```python
from build123d import *

# Parameters (mm, degrees)
EXTRUDE_1_DEPTH             = 38
SKETCH_3_R                  = 4.35
EXTRUDE_2_DEPTH             = 288
EXTRUDE_3_DEPTH             = 38
SKETCH_5_W                  = 42
SKETCH_5_H                  = 27.5
PATTERN_LINEAR_1_COUNT      = 2
PATTERN_LINEAR_1_PITCH      = 89
PATTERN_LINEAR_1_COUNT_DIR2 = 2
PATTERN_LINEAR_1_PITCH_DIR2 = 89
PATTERN_LINEAR_2_COUNT      = 2
PATTERN_LINEAR_2_PITCH      = 89
PATTERN_LINEAR_2_COUNT_DIR2 = 2
PATTERN_LINEAR_2_PITCH_DIR2 = 89


with BuildPart() as part:
    # Sketch 1 → Extrude 1 (new body)
    with BuildSketch(Plane(origin=(0, 0, 0), x_dir=(0, 0, -1), z_dir=(1, 0, 0))):
        with BuildLine():
            Line((-52, -57), (52, -57))
            ThreePointArc((52, -57), (55.535533906, -55.535533906), (57, -52))
            Line((57, -52), (57, 52))
            ThreePointArc((57, 52), (55.535533906, 55.535533906), (52, 57))
            Line((52, 57), (-52, 57))
            ThreePointArc((-52, 57), (-55.535533906, 55.535533906), (-57, 52))
            Line((-57, 52), (-57, -52))
            ThreePointArc((-57, -52), (-55.535533906, -55.535533906), (-52, -57))
        make_face()
    extrude(amount=EXTRUDE_1_DEPTH)

    # Sketch 2 → Revolve 1 (revolve)
    with BuildSketch(Plane(origin=(0, 0, 0), x_dir=(1, 0, 0), z_dir=(0, 1, 0))):
        with BuildLine():
            Line((-20, 0), (-20, 23))
            ThreePointArc((-20, 23), (-19.707106781, 23.707106781), (-19, 24))
            Line((-19, 24), (-5, 24))
            Line((-5, 24), (-5, 26.5))
            ThreePointArc((-5, 26.5), (-4.707106781, 27.207106781), (-4, 27.5))
            Line((-4, 27.5), (38, 27.5))
            Line((38, 27.5), (38, 0))
            Line((38, 0), (-20, 0))
        make_face()
    revolve(axis=Axis((38, 0, 0), (-1, 0, 0)))

    # Sketch 3 → Extrude 2 (add)
    with BuildSketch(Plane(origin=(38, 0, 0), x_dir=(0, 0, -1), z_dir=(1, 0, 0))):
        with BuildLine():
            Line((-43.968530717, -33.361928999), (-51.303300859, -40.696699141))
            ThreePointArc((-51.303300859, -40.696699141), (-51.303300859, -51.303300859), (-40.696699141, -51.303300859))
            Line((-40.696699141, -51.303300859), (-33.361928999, -43.968530717))
            ThreePointArc((-33.361928999, -43.968530717), (-32.119521583, -43.390137282), (-30.796446235, -43.747330196))
            ThreePointArc((-30.796446235, -43.747330196), (1.08e-07, -53.5), (30.796446412, -43.747330071))
            ThreePointArc((30.796446412, -43.747330071), (32.119521691, -43.390137291), (33.361928999, -43.968530717))
            Line((33.361928999, -43.968530717), (40.696699141, -51.303300859))
            ThreePointArc((40.696699141, -51.303300859), (51.303300859, -51.303300859), (51.303300859, -40.696699141))
            Line((51.303300859, -40.696699141), (43.968530717, -33.361928999))
            ThreePointArc((43.968530717, -33.361928999), (43.390137282, -32.119521583), (43.747330196, -30.796446235))
            ThreePointArc((43.747330196, -30.796446235), (53.5, 1.08e-07), (43.747330071, 30.796446412))
            ThreePointArc((43.747330071, 30.796446412), (43.390137291, 32.119521691), (43.968530717, 33.361928999))
            Line((43.968530717, 33.361928999), (51.303300859, 40.696699141))
            ThreePointArc((51.303300859, 40.696699141), (51.303300859, 51.303300859), (40.696699141, 51.303300859))
            Line((40.696699141, 51.303300859), (33.361928999, 43.968530717))
            ThreePointArc((33.361928999, 43.968530717), (32.119521583, 43.390137282), (30.796446235, 43.747330196))
            ThreePointArc((30.796446235, 43.747330196), (-1.08e-07, 53.5), (-30.796446412, 43.747330071))
            ThreePointArc((-30.796446412, 43.747330071), (-32.119521691, 43.390137291), (-33.361928999, 43.968530717))
            Line((-33.361928999, 43.968530717), (-40.696699141, 51.303300859))
            ThreePointArc((-40.696699141, 51.303300859), (-51.303300859, 51.303300859), (-51.303300859, 40.696699141))
            Line((-51.303300859, 40.696699141), (-43.968530717, 33.361928999))
            ThreePointArc((-43.968530717, 33.361928999), (-43.390137282, 32.119521583), (-43.747330196, 30.796446235))
            ThreePointArc((-43.747330196, 30.796446235), (-53.5, -1.08e-07), (-43.747330071, -30.796446412))
            ThreePointArc((-43.747330071, -30.796446412), (-43.390137291, -32.119521691), (-43.968530717, -33.361928999))
        make_face()
        with Locations((44.5, 44.5)):
            Circle(SKETCH_3_R, mode=Mode.SUBTRACT)
        with Locations((44.5, -44.5)):
            Circle(SKETCH_3_R, mode=Mode.SUBTRACT)
        with Locations((-44.5, 44.5)):
            Circle(SKETCH_3_R, mode=Mode.SUBTRACT)
        with Locations((-44.5, -44.5)):
            Circle(SKETCH_3_R, mode=Mode.SUBTRACT)
    extrude(amount=EXTRUDE_2_DEPTH)

    # Sketch 4 → Extrude 3 (add)
    with BuildSketch(Plane(origin=(364, 0, 0), x_dir=(0, 0, -1), z_dir=(1, 0, 0))):
        with BuildLine():
            Line((-52, -57), (52, -57))
            ThreePointArc((52, -57), (55.535533906, -55.535533906), (57, -52))
            Line((57, -52), (57, 52))
            ThreePointArc((57, 52), (55.535533906, 55.535533906), (52, 57))
            Line((52, 57), (-52, 57))
            ThreePointArc((-52, 57), (-55.535533906, 55.535533906), (-57, 52))
            Line((-57, 52), (-57, -52))
            ThreePointArc((-57, -52), (-55.535533906, -55.535533906), (-52, -57))
        make_face()
    extrude(amount=-EXTRUDE_3_DEPTH)

    # Sketch 5 → Revolve 2 (revolve)
    with BuildSketch(Plane.XY):
        with Locations((347, 13.75)):
            Rectangle(SKETCH_5_W, SKETCH_5_H)
    revolve(axis=Axis((368, 0, 0), (-1, 0, 0)))

    # Sketch 6 → Cut-Revolve 1 (revolve, cut)
    with BuildSketch(Plane(origin=(0, 17, 0), x_dir=(1, 0, 0), z_dir=(0, 1, 0))):
        Polygon((19, -57), (8.5225, -57), (9.6845, -55.838), (9.6845, -35), (19, -29.621693567), align=None)
    revolve(axis=Axis((19, 17, 29.621693567), (0, 0, 1)), mode=Mode.SUBTRACT)

    # Sketch 7 → Cut-Revolve 2 (revolve, cut)
    with BuildSketch(Plane(origin=(0, 17, 0), x_dir=(1, 0, 0), z_dir=(0, 1, 0))):
        Polygon((345, -57), (334.5225, -57), (335.6845, -55.838), (335.6845, -35), (345, -29.621693567), align=None)
    revolve(axis=Axis((345, 17, 29.621693567), (0, 0, 1)), mode=Mode.SUBTRACT)

    # Sketch 8 → Cut-Revolve 3 (revolve, cut)
    with BuildSketch(Plane(origin=(0, -15, 0), x_dir=(1, 0, 0), z_dir=(0, 1, 0))):
        Polygon((28.5, -57), (22.95, -57), (23.45, -56.5), (23.45, -53.5), (23.95, -53.5), (23.95, -56), (24.45, -56.5), (26, -56.5), (26, -53.5), (28.5, -53.5), align=None)
    revolve(axis=Axis((28.5, -15, 53.5), (0, 0, 1)), mode=Mode.SUBTRACT)

    # Sketch 9 → Cut-Revolve 4 (revolve, cut)
    with BuildSketch(Plane(origin=(0, -15, 0), x_dir=(1, 0, 0), z_dir=(0, 1, 0))):
        Polygon((335.5, -57), (329.95, -57), (330.45, -56.5), (330.45, -53.5), (330.95, -53.5), (330.95, -56), (331.45, -56.5), (333, -56.5), (333, -53.5), (335.5, -53.5), align=None)
    revolve(axis=Axis((335.5, -15, 53.5), (0, 0, 1)), mode=Mode.SUBTRACT)

    # Sketch 10 → Cut-Revolve 5 (revolve, cut)
    with BuildSketch(Plane.XY.offset(-44.5)):
        Polygon((22, -44.5), (22, -48.688), (8.812, -48.688), (8, -49.5), (8, -52.45), (0, -52.45), (0, -44.5), align=None)
    cut_revolve_5 = revolve(axis=Axis((0, -44.5, -44.5), (1, 0, 0)), mode=Mode.SUBTRACT)

    # Pattern Linear 1: Cut-Revolve 5 2 × 2
    with Locations(*[(0, i * PATTERN_LINEAR_1_PITCH, j * PATTERN_LINEAR_1_PITCH_DIR2) for i in range(PATTERN_LINEAR_1_COUNT) for j in range(PATTERN_LINEAR_1_COUNT_DIR2) if (i, j) != (0, 0)]):
        add(cut_revolve_5, mode=Mode.SUBTRACT)

    # Sketch 12 → Cut-Revolve 6 (revolve, cut)
    with BuildSketch(Plane.XY.offset(-44.5)):
        Polygon((364, -44.5), (364, -52.45), (356, -52.45), (356, -49.5), (355.188, -48.688), (342, -48.688), (342, -44.5), align=None)
    cut_revolve_6 = revolve(axis=Axis((342, -44.5, -44.5), (1, 0, 0)), mode=Mode.SUBTRACT)

    # Pattern Linear 2: Cut-Revolve 6 2 × 2
    with Locations(*[(0, i * PATTERN_LINEAR_2_PITCH, j * PATTERN_LINEAR_2_PITCH_DIR2) for i in range(PATTERN_LINEAR_2_COUNT) for j in range(PATTERN_LINEAR_2_COUNT_DIR2) if (i, j) != (0, 0)]):
        add(cut_revolve_6, mode=Mode.SUBTRACT)

    # Sketch 14 → Cut-Revolve 7 (revolve, cut)
    with BuildSketch(Plane.XY):
        Polygon((-20, 0), (-20, 15), (-1, 15), (-1, 18.2), (35, 18.2), (35, 50), (329, 50), (329, 18.2), (365, 18.2), (365, 0), align=None)
    revolve(axis=Axis((365, 0, 0), (-1, 0, 0)), mode=Mode.SUBTRACT)


solid = part.part
```
Build history of the part. All positions in model axes, mm. A direction names the side the tool comes from. Give positions to 0.01 mm unless a question says otherwise; leave off trailing zeros. One line per question, with ' | ' between items.
Q1. Cut at A-A, the plane x = 184. Count the separate pieces of the cut face and the enclosed holes in it, plus the area to 3 significant figures.
Filled sheet:
separate pieces: 1 | enclosed holes: 5 | area: 1,960 mm²
Q2. Drill centre lines: line 1 along Z through (x, y) = (346, 44.5); line 2 along Z through (x, y) = (362.25, -44.5); line 3 along Y through (x, z) = (2, -44). Where is each one in solid material? Low to high. Write a range as [from, to].
Filled sheet:
line 1: z = [-57, -48.69], [-40.31, 40.31], [48.69, 57] | line 2: z = [-57, -52.45], [-36.55, 36.55], [52.45, 57] | line 3: y = [-57, -52.43], [-36.57, 36.57], [52.43, 57]
Q3. Tool access for faces 1 (the cylindrical face through (32.11, -12.23, 54.77)), 2 (the flat face through (356, -44, -39)), 3 (the cylindrical face through (15.314, -48.495, -45.758)), 4 (the flat face through (179.984, 47.687, -37.081)), 5 (the cylindrical face through (179.984, 47.44, -41.294)): list every direction of +Z, -Z, +X, -X, +Y, -Y with a clear straight run to the whole face (end or side of a thin tool).
Filled sheet:
face 1: +Z | face 2: +X | face 3: -X | face 4: +Y | face 5: none
Q4. Drop flat-ended pins along their axis: pin 1 (4.5 mm diameter, centred on y = 44, z = 44, fed in from +X); pin 2 (12.5 mm diameter, centred on y = -44.5, z = -44.5, fed in from -X); pin 3 (2 mm diameter, centred on y = 29, z = -27, fed in from +X). Give the stop position or say it passes through.
Filled sheet:
pin 1: stops at x = 342 | pin 2: stops at x = 8 | pin 3: stops at x = 364
Q5. Pull direction Z, two halves, no side cores. Call faces 6 (the flat face through (345, 1, 57)), 7 (the flat face through (342, 45, -45)), 8 (the flat face through (19, -1, -57)): pulls with the +Z half, pulls with the -Z half, needs draft (parallel to the pull), parting line crosses it, or undercut.
Filled sheet:
face 6: pulls with the +Z half | face 7: undercut | face 8: pulls with the -Z half
